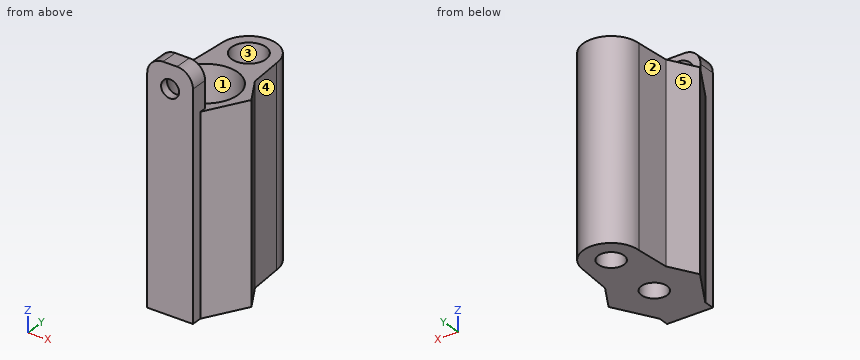
```python
from build123d import *

# Parameters (mm, degrees)
SKETCH1_R           = 2.44
BOSS_EXTRUDE2_DEPTH = 37
SKETCH8_R           = 3.25
SKETCH8_R_2         = 6.075
CUT_EXTRUDE1_DEPTH  = 33
BOSS_EXTRUDE4_DEPTH = 37
SKETCH18_W          = 8.660254038
SKETCH18_H          = 37
BOSS_EXTRUDE5_DEPTH = 2
SKETCH19_W          = 8.660254038
SKETCH19_H          = 3.245908706
BOSS_EXTRUDE6_DEPTH = 8
FILLET4_R           = 3


with BuildPart() as part:
    # Sketch1 → Boss-Extrude2 (new body)
    with BuildSketch(Plane.XY):
        with BuildLine():
            ThreePointArc((3.987455097, 4.316546763), (0, 8), (-3.987455097, 4.316546763))
            Line((-3.987455097, 4.316546763), (-4.330127019, 0))
            Line((-4.330127019, 0), (-8.660254038, -7.5))
            Line((-8.660254038, -7.5), (-4.330127019, -15))
            Line((-4.330127019, -15), (4.330127019, -15))
            Line((4.330127019, -15), (8.660254038, -7.5))
            Line((8.660254038, -7.5), (4.330127019, 0))
            Line((4.330127019, 0), (3.987455097, 4.316546763))
        make_face()
        with Locations((0, 4)):
            Circle(SKETCH1_R, mode=Mode.SUBTRACT)
        with Locations((0, -7.5)):
            Circle(SKETCH1_R, mode=Mode.SUBTRACT)
    extrude(amount=BOSS_EXTRUDE2_DEPTH)

    # Sketch8 → Cut-Extrude1 (cut)
    with BuildSketch(Plane.XY.offset(37)):
        with Locations((0, 4)):
            Circle(SKETCH8_R)
        with Locations((0, -7.5)):
            Circle(SKETCH8_R_2)
    extrude(amount=-CUT_EXTRUDE1_DEPTH, mode=Mode.SUBTRACT)

    # Sketch15 → Boss-Extrude4 (add)
    with BuildSketch(Plane.XY.offset(37)):
        with BuildLine():
            ThreePointArc((5.25, 4), (0, 9.25), (-5.25, 4))
            ThreePointArc((-5.25, 4), (-4.995467041, 2.385128786), (-4.256548938, 0.926843456))
            Line((-4.256548938, 0.926843456), (-3.987455097, 4.316546763))
            ThreePointArc((-3.987455097, 4.316546763), (0, 8), (3.987455097, 4.316546763))
            Line((3.987455097, 4.316546763), (4.256548938, 0.926843456))
            ThreePointArc((4.256548938, 0.926843456), (4.995467041, 2.385128786), (5.25, 4))
        make_face()
        with BuildLine():
            ThreePointArc((-4.256548938, 0.926843456), (-4.995467041, 2.385128786), (-5.25, 4))
            Line((-5.25, 4), (-5.753496857, -2.465348878))
            Line((-5.753496857, -2.465348878), (-4.330127019, 0))
            Line((-4.330127019, 0), (-4.256548938, 0.926843456))
        make_face()
        with BuildLine():
            Line((5.753496857, -2.465348878), (5.25, 4))
            ThreePointArc((5.25, 4), (4.995467041, 2.385128786), (4.256548938, 0.926843456))
            Line((4.256548938, 0.926843456), (4.330127019, 0))
            Line((4.330127019, 0), (5.753496857, -2.465348878))
        make_face()
    extrude(amount=-BOSS_EXTRUDE4_DEPTH)

    # Sketch18 → Boss-Extrude5 (add)
    with BuildSketch(Plane.XZ.offset(15)):
        with Locations((0, 18.5)):
            Rectangle(SKETCH18_W, SKETCH18_H)
    extrude(amount=BOSS_EXTRUDE5_DEPTH)

    # Sketch19 → Boss-Extrude6 (add)
    with BuildSketch(Plane.XY.offset(37)):
        with Locations((0, -15.377045647)):
            Rectangle(SKETCH19_W, SKETCH19_H)
    extrude(amount=BOSS_EXTRUDE6_DEPTH)

    # Fillet4
    fillet4_edges = [part.edges().sort_by_distance(p)[0] for p in [
        (-4.330127019, -15.377045647, 45),
        (4.330127019, -15.377045647, 45),
    ]]
    fillet(fillet4_edges, radius=FILLET4_R)

    # Sketch21 → CSK for M3 Hex Socket Countersunk Cap Screw1 (revolve, cut)
    with BuildSketch(Plane(origin=(0, -13.754091294, 40.565360139), x_dir=(0, 0, 1), z_dir=(1, 0, 0))):
        Polygon((0, 0), (0, 3.245908706), (1.7, 3.245908706), (1.7, 1.66), (3.36, 0), align=None)
    revolve(axis=Axis((0, -7.404091294, 40.565360139), (0, -1, 0)), mode=Mode.SUBTRACT)


solid = part.part
```
Could you check a few things on this model? Use its own coordinates, in mm. Face numbers are marked on the shaded views. A direction names the side the tool comes from. Round coordinates to 2 decimals unless told otherwise and drop trailing zeros. Loops run counter-clockwise (first coordinate to the right, second up) from the corner with the lowest first, then second, coordinate; pieces in that order, holes last. Notation, with made-up numbers: M -18.75,59.25 L -8.75,59.25 A12 cw -8.75,82.25 Z; hole C -11,46.5 d1. An arc over 180 degrees is marked long. Answer as CSV lines item,"result".
1) For pin 1 Ø5 at (y, z) = (-3.5, 18) entering from +X; pin 2 Ø3 at (x, y) = (1.5, 2.5) entering from +Z; pin 3 Ø1.6 at (y, z) = (-16, 20) entering from +X, each with a flat end and sliding along its axis, tell me the tip position at first contact or that it passes through.
From the geometry:
pin 1,"x = 7.79"
pin 2,"z = 37"
pin 3,"x = 4.33"
2) Imagine slicing it at B-B on z = 31.5. Count the separate pieces of the cut face and the enclosed holes in it, and give its area (3 significant figures).
From the geometry:
separate pieces,"1"
enclosed holes,"2"
area,"153 mm^2"
3) Imagine slicing it at A-A on x = 0. List the corners of the cut face in (y, z) for me (3 decimals), and give its area (3 significant figures).
From the geometry:
outline,"M -17,0 L -9.94,0 L -9.94,4 L -13.575,4 L -13.575,37 L -13.754,37 L -13.754,37.205 L -15.414,38.865 L -17,38.865 Z; M -17,42.265 L -15.414,42.265 L -13.754,43.925 L -13.754,45 L -17,45 Z; M -5.06,0 L 1.56,0 L 1.56,4 L 0.75,4 L 0.75,37 L -1.425,37 L -1.425,4 L -5.06,4 Z; M 6.44,0 L 9.25,0 L 9.25,37 L 7.25,37 L 7.25,4 L 6.44,4 Z"
area,"329 mm^2"
4) If I drill on probe 1 along Y at (x, z) = (0, 26) (3 decimals); probe 2 along X at (y, z) = (4.25, 19); probe 3 along X at (y, z) = (-7.5, 2.5), over which ranges is the centre line in solid material (lowest first)?
From the geometry:
probe 1,"-17 to -13.575, -1.425 to 0.75, 7.25 to 9.25"
probe 2,"-5.24 to -3.24, 3.24 to 5.24"
probe 3,"-8.66 to -2.44, 2.44 to 8.66"
5) Which directions (+Z, -Z, +X, -X, +Y, -Y) give clear straight access to the entire face, cutting with the end or side of a thin tool? Please do the marked faces 1 and 2.
From the geometry:
face 1,"+Z"
face 2,"+Z, -Z, -X, +Y"
6) We'd pull the mould along X, two halves only. Please class the marked faces 3, 4 and 5: released by +X, released by -X, zero draft, split by the parting line, or undercut.
From the geometry:
face 3,"undercut"
face 4,"released by +X"
face 5,"released by -X"
